from build123d import *

# Parameters (mm, degrees)
SKETCH1_W           = 45
SKETCH1_H           = 21.21
BOSS_EXTRUDE1_DEPTH = 1.5875
SKETCH2_W           = 45
SKETCH2_H           = 1.5875
BOSS_EXTRUDE2_DEPTH = 20.62570344
CUT_EXTRUDE3_DEPTH  = 55.482020035
CUT_EXTRUDE4_DEPTH  = 53.373835995


with BuildPart() as part:
    # Sketch1 → Boss-Extrude1 (new body)
    with BuildSketch(Plane.XY):
        with Locations((22.5, 10.605)):
            Rectangle(SKETCH1_W, SKETCH1_H)
    extrude(amount=BOSS_EXTRUDE1_DEPTH)

    # Sketch2 → Boss-Extrude2 (add)
    with BuildSketch(Plane.XY.offset(1.5875)):
        with Locations((22.5, 0.79375)):
            Rectangle(SKETCH2_W, SKETCH2_H)
    extrude(amount=BOSS_EXTRUDE2_DEPTH)

    # Sketch5 → Cut-Extrude3 (cut, through all)
    with BuildSketch(Plane(origin=(0, 0, 0), x_dir=(-1, 0, 0), z_dir=(0, 0, -1))):
        Polygon((-21.21, 21.21), (0, 0), (0, 21.21), align=None)
        Polygon((-45, 0), (-21.213203436, 0), (-42.423203436, 21.21), (-45, 21.21), align=None)
    extrude(amount=-CUT_EXTRUDE3_DEPTH, mode=Mode.SUBTRACT)

    # Sketch4 → Cut-Extrude4 (cut, through all)
    with BuildSketch(Plane(origin=(0, 0, 0), x_dir=(-1, 0, 0), z_dir=(0, 0, -1))):
        with BuildLine():
            ThreePointArc((-14.409101718, 5.3025), (-15.335076569, 6.688319299), (-16.96976189, 6.363160172))
            Line((-16.96976189, 6.363160172), (-14.848441546, 4.241839828))
            ThreePointArc((-14.848441546, 4.241839828), (-14.523282419, 4.728474851), (-14.409101718, 5.3025))
        make_face()
        with BuildLine():
            Line((-14.848441546, 4.241839828), (-16.96976189, 6.363160172))
            ThreePointArc((-16.96976189, 6.363160172), (-16.96976189, 4.241839828), (-14.848441546, 4.241839828))
        make_face()
        with BuildLine():
            ThreePointArc((-25.014101718, 15.9075), (-25.940076569, 17.293319299), (-27.57476189, 16.968160172))
            Line((-27.57476189, 16.968160172), (-25.453441546, 14.846839828))
            ThreePointArc((-25.453441546, 14.846839828), (-25.128282419, 15.333474851), (-25.014101718, 15.9075))
        make_face()
        with BuildLine():
            Line((-25.453441546, 14.846839828), (-27.57476189, 16.968160172))
            ThreePointArc((-27.57476189, 16.968160172), (-27.57476189, 14.846839828), (-25.453441546, 14.846839828))
        make_face()
    extrude(amount=-CUT_EXTRUDE4_DEPTH, mode=Mode.SUBTRACT)


solid = part.part
Could you check a few things on this model? Use its own coordinates, in mm. A direction names the side the tool comes from. Round coordinates to 2 decimals unless told otherwise and drop trailing zeros. Write each loop counter-clockwise with the first axis right and the second up, starting at its lowest first coordinate (ties: lowest second). Pieces come first, ordered by that corner, then holes. Notation, with made-up numbers: (65.25, 84.5) - (102.25, 84.5) arc R25 ccw to (102.25, 122.5) - close; hole circle Ø3 at (15, 73.25). An arc over 180 degrees is marked (long way). Use a Markdown table: item, result.
Q1. I want a section at A-A (x = 26.5). List the corners of the cut face in (y, z) for me.
Output values:
| item | result |
|---|---|
| outline | (5.29, 0) - (14.41, 0) - (14.41, 1.59) - (5.29, 1.59) - close; (17.41, 0) - (21.21, 0) - (21.21, 1.59) - (17.41, 1.59) - close |
Q2. I want a section at D-D (y = 11.5). List the corners of the cut face in (x, z) for me.
Output values:
| item | result |
|---|---|
| outline | (11.5, 0) - (32.71, 0) - (32.71, 1.59) - (11.5, 1.59) - close |
Q3. Please list where these lines run through material, in increasing order: L1, parallel to Y at x = 9.5, z = 13.25; L2, parallel to Y at x = 22.5, z = 3.75.
Output values:
| item | result |
|---|---|
| L1 | 0 to 1.59 |
| L2 | 1.29 to 1.59 |
Q4. For pin 1 (1 mm diameter, centred on x = 16, y = 17, fed in from -Z); pin 2 (10 mm diameter, centred on x = 14.5, y = 16, fed in from +Z); pin 3 (2 mm diameter, centred on x = 22.5, z = 9.5, fed in from +Y), each with a flat end and sliding along its axis, tell me the tip position at first contact or that it passes through.
Output values:
| item | result |
|---|---|
| pin 1 | through |
| pin 2 | z = 1.59 |
| pin 3 | y = 1.59 |
Q5. I want a section at C-C (z = 16). List the corners of the cut face in (x, y) for me.
Output values:
| item | result |
|---|---|
| outline | (0, 0) - (21.21, 0) - (22.8, 1.59) - (1.59, 1.59) - close |
Q6. For faces 1 (the flat face through (22, 12, 1.588)), 2 (the flat face through (10, 0, 11)), which set-ups out of +Z, -Z, +X, -X, +Y, -Y let a thin tool reach every point of the face, with its end or its side?
Output values:
| item | result |
|---|---|
| face 1 | +Z, +X, -X, +Y |
| face 2 | +Z, -Z, +X, -X, -Y |
Q7. I want a section at B-B (x = 6.5). List the corners of the cut face in (y, z) for me, plus the area to 3 significant figures.
Output values:
| item | result |
|---|---|
| outline | (0, 0) - (6.5, 0) - (6.5, 1.59) - (1.59, 1.59) - (1.59, 22.21) - (0, 22.21) - close |
| area | 43.1 mm2 |
